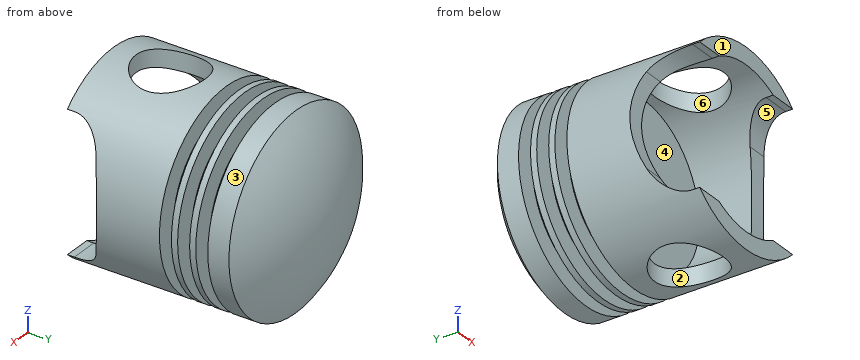
```python
from build123d import *

# Parameters (mm, degrees)
SKETCH1_R               = 26.45
BOSS_EXTRUDE1_DEPTH     = 50
CUT_EXTRUDE2_START      = -5.8
SKETCH2_OUTSIDE_W       = 72.896
SKETCH2_OUTSIDE_H       = 72.896
SKETCH2_OUTSIDE_R       = 21
CUT_EXTRUDE2_DEPTH      = 3.3
LPATTERN1_COUNT         = 3
LPATTERN1_PITCH         = 5
SKETCH5_R               = 21.804512809
CUT_EXTRUDE4_DEPTH      = 28
DOME1_FACE_RADIUS       = 26.45
DOME1_HEIGHT            = 9
CUT_EXTRUDE5_DEPTH      = 70.858464054
CUT_EXTRUDE5_DEPTH_BACK = 70.858464054
SKETCH6_R               = 9.520481224
CUT_EXTRUDE6_DEPTH      = 70.85846413
CUT_EXTRUDE6_DEPTH_BACK = 70.85846413
FILLET1_R               = 10
FILLET2_R               = 10


with BuildPart() as part:
    # Sketch1 → Boss-Extrude1 (new body)
    with BuildSketch(Plane(origin=(0, 0, 0), x_dir=(1, 0, 0), z_dir=(0, 1, 0))):
        with Locations(Location((0, 0, 0), (0, 0, 270))):
            Circle(SKETCH1_R)
    extrude(amount=BOSS_EXTRUDE1_DEPTH)

    # Sketch2 outside → Cut-Extrude2 (cut)
    with BuildSketch(Plane(origin=(0, 50, 0), x_dir=(1, 0, 0), z_dir=(0, 1, 0)).offset(CUT_EXTRUDE2_START)):
        Rectangle(SKETCH2_OUTSIDE_W, SKETCH2_OUTSIDE_H)
        with Locations(Location((0, 0, 0), (0, 0, 270))):
            Circle(SKETCH2_OUTSIDE_R, mode=Mode.SUBTRACT)
    cut_extrude2 = extrude(amount=-CUT_EXTRUDE2_DEPTH, mode=Mode.SUBTRACT)

    # LPattern1: Cut-Extrude2 ×3
    with Locations(*[(0, -i * LPATTERN1_PITCH, 0) for i in range(1, LPATTERN1_COUNT)]):
        add(cut_extrude2, mode=Mode.SUBTRACT)

    # Sketch5 → Cut-Extrude4 (cut)
    with BuildSketch(Plane.XZ):
        with Locations(Location((0, 0, 0), (0, 0, 270))):
            Circle(SKETCH5_R)
    extrude(amount=-CUT_EXTRUDE4_DEPTH, mode=Mode.SUBTRACT)

    # Dome1: a dome of height H over a round flat face of radius A is a cap of a sphere of radius (A * A + H * H) / (2 * H)
    dome1_r = (DOME1_FACE_RADIUS * DOME1_FACE_RADIUS + DOME1_HEIGHT * DOME1_HEIGHT) / (2 * DOME1_HEIGHT)
    dome1_base = Plane((0, 50, 0), z_dir=(0, 1, 0))
    with Locations(dome1_base.offset(DOME1_HEIGHT - dome1_r)):
        dome1_ball = Sphere(dome1_r, mode=Mode.PRIVATE)
    add(split(dome1_ball, bisect_by=dome1_base, keep=Keep.TOP, mode=Mode.PRIVATE))

    # Sketch6 → Cut-Extrude5 (cut, two sides: drawn at the far end of the back side and taken through both)
    with BuildSketch(Plane.XY.offset(-CUT_EXTRUDE5_DEPTH_BACK)):
        with Locations((0, 15.633194444)):
            Circle(SKETCH6_R)
    extrude(amount=CUT_EXTRUDE5_DEPTH + CUT_EXTRUDE5_DEPTH_BACK, mode=Mode.SUBTRACT)

    # Sketch8 → Cut-Extrude6 (cut, two sides: drawn at the far end of the back side and taken through both)
    with BuildSketch(Plane(origin=(0, 0, 0), x_dir=(0, 0, -1), z_dir=(1, 0, 0)).offset(-CUT_EXTRUDE6_DEPTH_BACK)):
        with BuildLine():
            Line((-19, 0), (-19, 8))
            ThreePointArc((-19, 8), (0, 13.606123087), (19, 8))
            Line((19, 8), (19, 0))
            Line((19, 0), (-19, 0))
        make_face()
    extrude(amount=CUT_EXTRUDE6_DEPTH + CUT_EXTRUDE6_DEPTH_BACK, mode=Mode.SUBTRACT)

    # Fillet1
    fillet1_edges = [part.edges().sort_by_distance(p)[0] for p in [
        (14.549333798, 8, -19),
        (14.549333798, 8, 19),
    ]]
    fillet(fillet1_edges, radius=FILLET1_R)

    # Fillet2
    fillet2_edges = [part.edges().sort_by_distance(p)[0] for p in [
        (-14.549333798, 8, 19),
        (-14.549333798, 8, -19),
    ]]
    fillet(fillet2_edges, radius=FILLET2_R)


solid = part.part
```
For this review, take the finished solid that the model builds, in its own axes (mm). Face numbers are marked on the shaded views. A direction names the side the tool comes from. Round coordinates to 2 decimals unless told otherwise and drop trailing zeros. Write each loop counter-clockwise with the first axis right and the second up, starting at its lowest first coordinate (ties: lowest second). Pieces come first, ordered by that corner, then holes. Notation, with made-up numbers: M 81.5,69 L 91.5,69 A12 ccw 91.5,83 Z; hole C -18,63 d1. An arc over 180 degrees is marked long. One line per item, written item: value. Start each with the question number.
(1) Machinability: for the marked faces 4, 5 and 6, which of the approach directions +Z, -Z, +X, -X, +Y, -Y give a long, thin tool a straight path to every point of the face, cutting with its end or side? Answer none if there is none.
(2) Wall thickness on line 1 (Y direction, x = -15, z = -15); line 2 (Y direction, x = 0, z = -22); line 3 (X direction, y = 7, z = 19): over which ranges is each line inside the solid? List them lowest first.
(3) Insertion check: pin 1 (17 mm diameter, centred on x = 0, y = 15.63, fed in from +Z); pin 2 (1.5 mm diameter, centred on y = 19.5, z = 18.5, fed in from +X); pin 3 (16 mm diameter, centred on x = 6.5, z = 1, fed in from -Y); pin 4 (16 mm diameter, centred on x = 13, z = -9.5, fed in from +Y). Each pin has a flat end and moves straight along its axis. Give the tip position at first contact, or say it passes through.
(4) The part is to be moulded in two halves that separate along X. For the marked faces 1, 2 and 3, say which applies: released by +X, released by -X, zero draft, split by the parting line, or undercut.
(5) We need section D-D (y = 49). Give the boundary of the cut face in (x, z), and give its area (3 significant figures).
(6) We need section A-A (y = 8.5). Give the boundary of the cut face in (x, z).
(7) We need section B-B (x = 0). Count the separate pieces of the cut face and the enclosed holes in it, and give its area (3 significant figures).
Result:
1. face 4: -Y
1. face 5: +X, -X, -Y
1. face 6: +Z, -Z
2. line 1: 28 to 30.9, 34.2 to 35.9, 39.2 to 40.9, 44.2 to 53.46
2. line 2: 0 to 6.11, 25.15 to 30.9, 34.2 to 35.9, 39.2 to 40.9, 44.2 to 53.01
2. line 3: -18.4 to -10.7, 10.7 to 18.4
3. pin 1: through
3. pin 2: x = 19.61
3. pin 3: y = 28
3. pin 4: y = 58.24
4. face 1: zero draft
4. face 2: undercut
4. face 3: split by the parting line
5. outline: C 0,0 d52.9
5. area: 2,200 mm²
6. outline: M -20.64,-16.54 A26.45 ccw -6.31,-25.69 L -6.31,-20.87 A21.8 cw -14.21,-16.54 Z; M -20.64,16.54 L -14.21,16.54 A21.8 cw -6.31,20.87 L -6.31,25.69 A26.45 ccw Z; M 6.31,-25.69 A26.45 ccw 20.64,-16.54 L 14.21,-16.54 A21.8 cw 6.31,-20.87 Z; M 6.31,20.87 A21.8 cw 14.21,16.54 L 20.64,16.54 A26.45 ccw 6.31,25.69 Z
7. separate pieces: 3
7. enclosed holes: 0
7. area: 1,460 mm²
